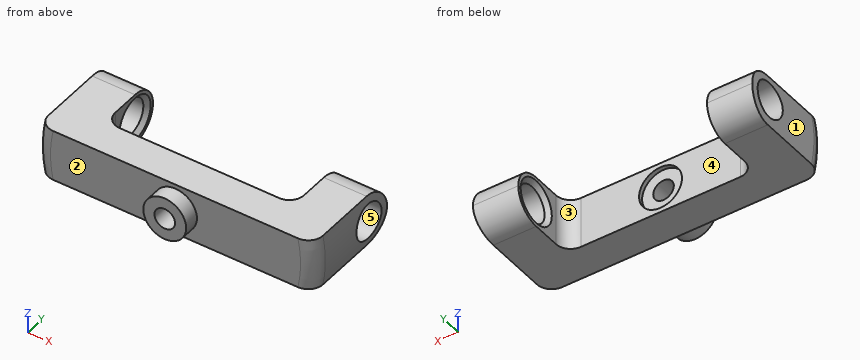
```python
from build123d import *

# Parameters (mm, degrees)
SKETCH1_W               = 5
SKETCH1_H               = 6
SKETCH1_W_2             = 22
BOSS_EXTRUDE1_DEPTH     = 4
BOSS_EXTRUDE2_START     = 4
SKETCH1_3_W             = 5
SKETCH1_3_H             = 6
BOSS_EXTRUDE2_DEPTH     = 8
CUT_EXTRUDE1_DEPTH      = 30.952196132
CUT_EXTRUDE1_DEPTH_BACK = 30.952196132
SKETCH2_R               = 2.1
SKETCH4_R               = 2.5
BOSS_EXTRUDE3_DEPTH     = 1.8
CUT_EXTRUDE2_DEPTH      = 22.550870206
CUT_EXTRUDE2_DEPTH_BACK = 22.550870206
SKETCH5_R               = 1.2
SKETCH6_R               = 2.5
CUT_EXTRUDE3_DEPTH      = 0.5
CHAMFER1_SIZE           = 0.5
FILLET1_R               = 1.7


with BuildPart() as part:
    # Sketch1 → Boss-Extrude1 (new body)
    with BuildSketch(Plane(origin=(0, 0, 0), x_dir=(1, 0, 0), z_dir=(0, 1, 0))):
        with Locations((-13.5, 0)):
            Rectangle(SKETCH1_W, SKETCH1_H)
        Rectangle(SKETCH1_W_2, SKETCH1_H)
        with Locations((13.5, 0)):
            Rectangle(SKETCH1_W, SKETCH1_H)
        with BuildLine():
            Line((-16, -3), (-16, 3))
            ThreePointArc((-16, 3), (-16.278820596, 0), (-16, -3))
        make_face()
        with BuildLine():
            ThreePointArc((16.278820596, 0), (16.208965568, 1.506464481), (16, 3))
            Line((16, 3), (16, -3))
            ThreePointArc((16, -3), (16.208965568, -1.506464481), (16.278820596, 0))
        make_face()
    extrude(amount=BOSS_EXTRUDE1_DEPTH)

    # Sketch1<3> → Boss-Extrude2 (add)
    with BuildSketch(Plane(origin=(0, 0, 0), x_dir=(1, 0, 0), z_dir=(0, 1, 0)).offset(BOSS_EXTRUDE2_START)):
        with Locations((-13.5, 0)):
            Rectangle(SKETCH1_3_W, SKETCH1_3_H)
        with BuildLine():
            Line((-16, -3), (-16, 3))
            ThreePointArc((-16, 3), (-16.278820596, 0), (-16, -3))
        make_face()
        with Locations((13.5, 0)):
            Rectangle(SKETCH1_3_W, SKETCH1_3_H)
        with BuildLine():
            ThreePointArc((16.278820596, 0), (16.208965568, 1.506464481), (16, 3))
            Line((16, 3), (16, -3))
            ThreePointArc((16, -3), (16.208965568, -1.506464481), (16.278820596, 0))
        make_face()
    extrude(amount=BOSS_EXTRUDE2_DEPTH)

    # Sketch2 → Cut-Extrude1 (cut, two sides: drawn at the far end of the back side and taken through both)
    with BuildSketch(Plane(origin=(-11, 0, 0), x_dir=(0, 0, -1), z_dir=(1, 0, 0)).offset(-CUT_EXTRUDE1_DEPTH_BACK)):
        with BuildLine():
            Line((3, 12), (0, 12))
            ThreePointArc((0, 12), (2.121320344, 11.121320344), (3, 9))
            Line((3, 9), (3, 12))
        make_face()
        with BuildLine():
            Line((-3, 12), (-3, 9))
            ThreePointArc((-3, 9), (-2.121320344, 11.121320344), (0, 12))
            Line((0, 12), (-3, 12))
        make_face()
        with Locations((0, 9)):
            Circle(SKETCH2_R)
    extrude(amount=CUT_EXTRUDE1_DEPTH + CUT_EXTRUDE1_DEPTH_BACK, mode=Mode.SUBTRACT)

    # Sketch4 → Boss-Extrude3 (add)
    with BuildSketch(Plane.XZ):
        with Locations(Location((0, 0, 0), (0, 0, 270))):
            Circle(SKETCH4_R)
    extrude(amount=BOSS_EXTRUDE3_DEPTH)

    # Sketch5 → Cut-Extrude2 (cut, two sides: drawn at the far end of the back side and taken through both)
    with BuildSketch(Plane.XZ.offset(1.8).offset(-CUT_EXTRUDE2_DEPTH_BACK)):
        with Locations(Location((0, 0, 0), (0, 0, 270))):
            Circle(SKETCH5_R)
    extrude(amount=CUT_EXTRUDE2_DEPTH + CUT_EXTRUDE2_DEPTH_BACK, mode=Mode.SUBTRACT)

    # Sketch6 → Cut-Extrude3 (cut)
    with BuildSketch(Plane(origin=(0, 4, 0), x_dir=(1, 0, 0), z_dir=(0, 1, 0))):
        with Locations(Location((0, 0, 0), (0, 0, 90))):
            Circle(SKETCH6_R)
    extrude(amount=-CUT_EXTRUDE3_DEPTH, mode=Mode.SUBTRACT)

    # Chamfer1
    chamfer1_edges = [part.edges().sort_by_distance(p)[0] for p in [
        (11, 9, 2.1),
        (-11, 9, 2.1),
    ]]
    chamfer(chamfer1_edges, length=CHAMFER1_SIZE)

    # Fillet1
    fillet1_edges = [part.edges().sort_by_distance(p)[0] for p in [
        (-11, 4, 0),
        (11, 4, 0),
        (-16.278820596, 0, 0),
        (16.278820596, 0, 0),
    ]]
    fillet(fillet1_edges, radius=FILLET1_R)


solid = part.part
```
The model under review builds one solid part; all positions refer to its coordinate system, in mm. Face numbers are marked on the shaded views. A direction names the side the tool comes from. Round coordinates to 2 decimals unless told otherwise and drop trailing zeros. Loops run counter-clockwise (first coordinate to the right, second up) from the corner with the lowest first, then second, coordinate; pieces in that order, holes last.
1) Consider section B-B on x = 12. State the section outline as (y, z) points, then the cut area to 3 significant figures.
Values follow:
outline: (0, -3) - (9, -3) arc R3 ccw to (9, 3) - (0, 3) - close; hole circle Ø4.2 at (9, 0)
area: 54.3 mm2
2) The part is to be moulded in two halves that separate along X. For the marked faces 1, 2 and 3, say which applies: pulls with the +X half, pulls with the -X half, needs draft (parallel to the pull), parting line crosses it, or undercut.
Values follow:
face 1: pulls with the -X half
face 2: needs draft
face 3: undercut
3) Consider section D-D on x = 7. State the section outline as (y, z) points.
Values follow:
outline: (0, -3) - (4, -3) - (4, 3) - (0, 3) - close
4) Wall thickness on line 1 along Y through (x, z) = (-13.4, 0); line 2 along Z through (x, y) = (-13.25, 9); line 3 along Y through (x, z) = (-2, 1): over which ranges is each line inside the solid? List them lowest first.
Values follow:
line 1: y = 0 to 6.9, 11.1 to 12
line 2: z = -3 to -2.1, 2.1 to 3
line 3: y = -1.8 to 3.5
5) Tool access review of the marked faces 4 and 5: name each direction out of +Z, -Z, +X, -X, +Y, -Y from which nothing blocks a thin tool from reaching the whole face with its end or side.
Values follow:
face 4: +Z, -Z, +Y
face 5: +X, -X
6) Clearance check with a flat-ended pin moving along its axis: P1, Ø2, axis at x = -6, z = 0, coming from the -Y side. State where the tip first meets the part, or that it passes through.
Values follow:
P1: stops at y = 0
7) Consider section C-C on y = 10. Give the number of separate pieces and of enclosed holes in the cut face, then the cut area to 3 significant figures.
Values follow:
separate pieces: 4
enclosed holes: 0
area: 19.5 mm2
8) Consider section A-A on x = 0. State the section outline as (y, z) points.
Values follow:
outline: (-1.8, -2.5) - (0, -2.5) - (0, -3) - (4, -3) - (4, -2.5) - (3.5, -2.5) - (3.5, -1.2) - (-1.8, -1.2) - close; (-1.8, 1.2) - (3.5, 1.2) - (3.5, 2.5) - (4, 2.5) - (4, 3) - (0, 3) - (0, 2.5) - (-1.8, 2.5) - close
